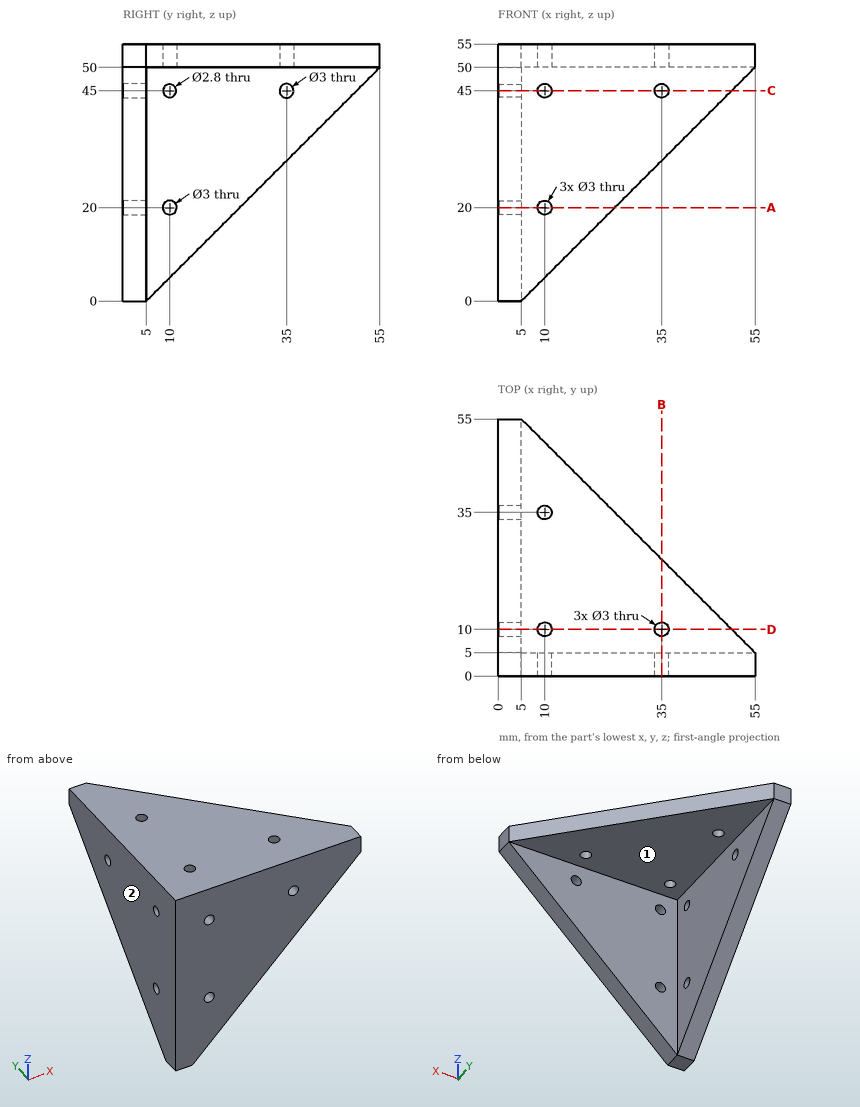
Study the drawing (mm; zero at the part's minimum x, y, z) and answer. A direction names the side the tool comes from. Coordinates: 2 decimals unless noted, no trailing zeros. Loops run counter-clockwise (first coordinate to the right, second up) from the corner with the lowest first, then second, coordinate; pieces in that order, holes last. Notation, with made-up numbers: (37, -36.5) -> (70, -36.5) arc R18 cw to (70, -21.5) -> close; hole circle Ø5 at (0.25, 35). An arc over 180 degrees is marked (long way). Answer in a Markdown table with one row per item. Add a question column.
1. For the marked faces 1 and 2, determine the directions among +Z, -Z, +X, -X, +Y, -Y from which every point of the face is accessible in a straight line to the end or side of a thin tool.
2. The part is cut by section A-A, the plane z = 20. Write down the section's boundary in (x, y), then the cut area to 3 significant figures.
3. Consider line 1 (Y direction, x = 10, z = 51); line 2 (Y direction, x = 1.4, z = 45); line 3 (Y direction, x = 36, z = 37.5). Determine where each line is inside the solid, lowest interval first. Write a range as [from, to].
4. The part is cut by section D-D, the plane y = 10. Write down the section's boundary in (x, z).
5. The part is cut by section B-B, the plane x = 35. Write down the section's boundary in (y, z), then the cut area to 3 significant figures.
6. The part is cut by section C-C, the plane z = 45. Write down the section's boundary in (x, y), then the cut area to 3 significant figures.
7. Flat-ended cylindrical pins translate along their axes: P1, Ø12, axis at y = 10, z = 15.5, coming from the -X side; P2, Ø4, axis at y = 25, z = 32, coming from the +X side. Find the tip coordinate at first contact, or state that the pin passes through.
Answer below:
| question | item | result |
|---|---|---|
| 1 | face 1 | -Z, +X, +Y |
| 1 | face 2 | +Z, -Z, -X, +Y, -Y |
| 2 | outline | (0, 0) -> (8.5, 0) -> (8.5, 5) -> (5, 5) -> (5, 8.5) -> (0, 8.5) -> close; (0, 11.5) -> (5, 11.5) -> (5, 25) -> (0, 25) -> close; (11.5, 0) -> (25, 0) -> (25, 5) -> (11.5, 5) -> close |
| 2 | area | 195 mm2 |
| 3 | line 1 | [0, 8.5], [11.5, 33.5], [36.5, 50] |
| 3 | line 2 | [0, 8.6], [11.4, 33.5], [36.5, 50] |
| 3 | line 3 | [0, 5] |
| 4 | outline | (0, 5) -> (5, 5) -> (5, 18.5) -> (0, 18.5) -> close; (0, 21.5) -> (5, 21.5) -> (5, 43.6) -> (0, 43.6) -> close; (0, 46.4) -> (5, 46.4) -> (5, 50) -> (8.5, 50) -> (8.5, 55) -> (0, 55) -> close; (11.5, 50) -> (33.5, 50) -> (33.5, 55) -> (11.5, 55) -> close; (36.5, 50) -> (50, 50) -> (50, 55) -> (36.5, 55) -> close |
| 5 | outline | (0, 30) -> (5, 30) -> (5, 43.5) -> (0, 43.5) -> close; (0, 46.5) -> (5, 46.5) -> (5, 50) -> (8.5, 50) -> (8.5, 55) -> (0, 55) -> close; (11.5, 50) -> (25, 50) -> (25, 55) -> (11.5, 55) -> close |
| 5 | area | 195 mm2 |
| 6 | outline | (0, 0) -> (8.5, 0) -> (8.5, 5) -> (5, 5) -> (5, 8.6) -> (0, 8.6) -> close; (0, 11.4) -> (5, 11.4) -> (5, 33.5) -> (0, 33.5) -> close; (0, 36.5) -> (5, 36.5) -> (5, 50) -> (0, 50) -> close; (11.5, 0) -> (33.5, 0) -> (33.5, 5) -> (11.5, 5) -> close; (36.5, 0) -> (50, 0) -> (50, 5) -> (36.5, 5) -> close |
| 6 | area | 416 mm2 |
| 7 | P1 | x = 0 |
| 7 | P2 | x = 5 |
